For this review, use the dimensioned drawing (mm, ordinates from the lowest corner) and the shaded views. A direction names the side the tool comes from. Give positions to 0.01 mm unless a question says otherwise; leave off trailing zeros. Order: outer loops, then holes, each group sorted by start corner. A loop starts at its lowest first (then second) coordinate and runs counter-clockwise, first axis right, second up. Notation, with made-up numbers: (30, 84) -> (36, 84) arc R26 cw to (36, 100) -> close; hole circle Ø10 at (85, -14.75). An arc over 180 degrees is marked (long way). Answer as a JSON object with one key per item and string values. Group by question number.
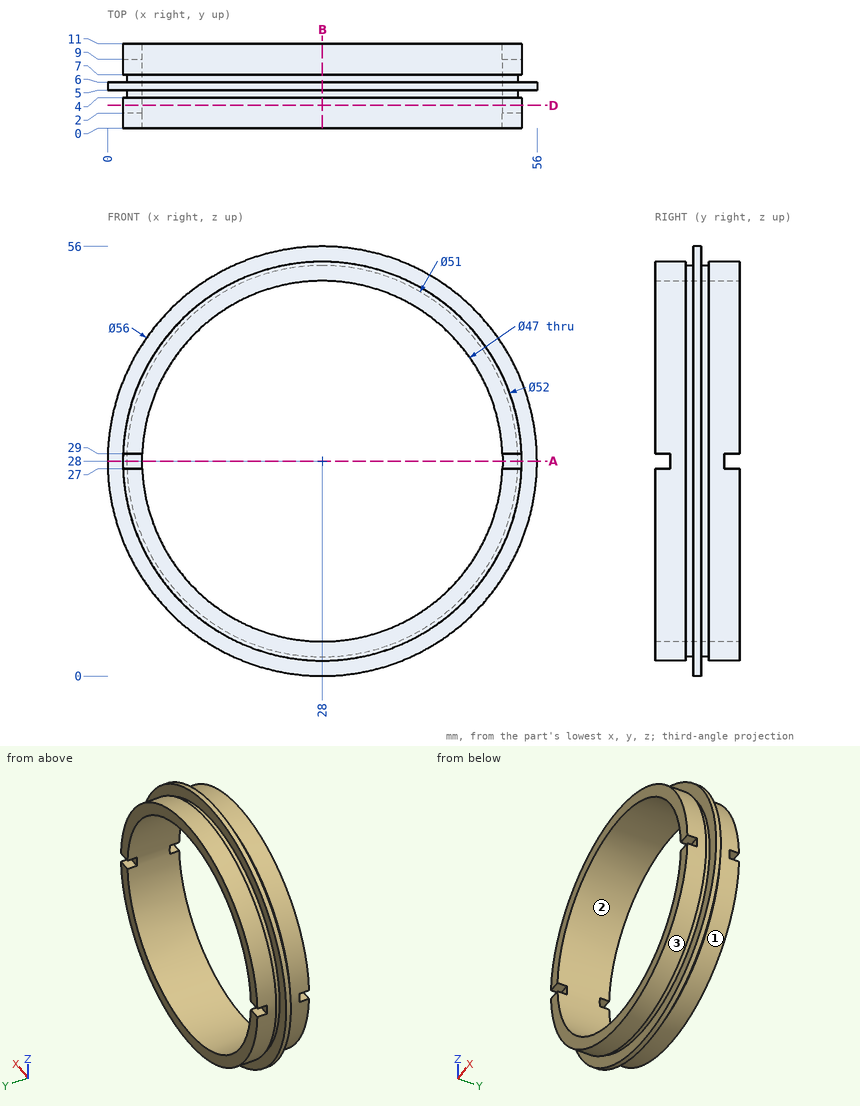
1. For pin 1 (2 mm diameter, centred on x = 53, y = 0.5, fed in from -Z); pin 2 (0.6 mm diameter, centred on x = 52.5, z = 28, fed in from -Y); pin 3 (1.6 mm diameter, centred on x = 3.5, y = 1.5, fed in from -Z), all flat-tipped, find the tip position at first contact; note any pin that passes through.
2. Machinability: for the marked faces 1, 2 and 3, which of the approach directions +Z, -Z, +X, -X, +Y, -Y give a long, thin tool a straight path to every point of the face, cutting with its end or side? Answer none if there is none.
3. Take a section at A-A on z = 28. Give the boundary of the cut face in (x, y), plus the area to 3 significant figures.
4. Take a section at D-D on y = 3. Give the boundary of the cut face in (x, z), plus the area to 3 significant figures.
5. Take a section at B-B on x = 28. Give the boundary of the cut face in (y, z), plus the area to 3 significant figures.
6. For probe 1 along X at (y, z) = (4.75, 28); probe 2 along X at (y, z) = (2.75, 48.5); probe 3 along Y at (x, z) = (11.5, 7), list the stretches that pass through material, from the lowest coordinate up. Write a range as [from, to].
Checks:
{
 "1": {"pin 1": "stops at z = 18", "pin 2": "stops at y = 2", "pin 3": "stops at z = 17.31"},
 "2": {"face 1": "+Y", "face 2": "+Y, -Y", "face 3": "-Y"},
 "3": {"outline": "(0, 5) -> (2.5, 5) -> (2.5, 4) -> (2, 4) -> (2, 2) -> (4.5, 2) -> (4.5, 9) -> (2, 9) -> (2, 7) -> (2.5, 7) -> (2.5, 6) -> (0, 6) -> close; (51.5, 2) -> (54, 2) -> (54, 4) -> (53.5, 4) -> (53.5, 5) -> (56, 5) -> (56, 6) -> (53.5, 6) -> (53.5, 7) -> (54, 7) -> (54, 9) -> (51.5, 9) -> close", "area": "37.0 mm2"},
 "4": {"outline": "circle Ø52 at (28, 28); hole circle Ø47 at (28, 28)", "area": "389 mm2"},
 "5": {"outline": "(0, 2) -> (4, 2) -> (4, 2.5) -> (5, 2.5) -> (5, 0) -> (6, 0) -> (6, 2.5) -> (7, 2.5) -> (7, 2) -> (11, 2) -> (11, 4.5) -> (0, 4.5) -> close; (0, 51.5) -> (11, 51.5) -> (11, 54) -> (7, 54) -> (7, 53.5) -> (6, 53.5) -> (6, 56) -> (5, 56) -> (5, 53.5) -> (4, 53.5) -> (4, 54) -> (0, 54) -> close", "area": "57.0 mm2"},
 "6": {"probe 1": "x = [2.5, 4.5], [51.5, 53.5]", "probe 2": "x = [12.01, 16.51], [39.49, 43.99]", "probe 3": "y = [5, 6]"}
}
